Read the model definition and answer for the solid it produces. Units are mm, in the model's axes. A direction names the side the tool comes from. Round coordinates to 2 decimals unless told otherwise and drop trailing zeros. Write each loop counter-clockwise with the first axis right and the second up, starting at its lowest first coordinate (ties: lowest second). Pieces come first, ordered by that corner, then holes. Notation, with made-up numbers: (25, 86.25) - (72, 86.25) arc R22 cw to (72, 93.25) - close; hole circle Ø10 at (8, 76). An arc over 180 degrees is marked (long way). Use one line per item in the form item = value. Start each with the question number.
1) Each of these flat-tipped pins is pushed along its axis until it touches: pin 1 (5 mm diameter, centred on x = -2.5, y = 7, fed in from -Z); pin 2 (0.5 mm diameter, centred on y = -3, z = -9, fed in from -X); pin 3 (2.5 mm diameter, centred on y = 5.5, z = -3.5, fed in from +X). Where does it stop, or does it pass through?
2) The part is cut by section B-B, the plane x = -4. Give the vertices of the cut face in (y, z) (3 decimals), plus the area to 3 significant figures.
3) The part is cut by section A-A, the plane y = -0.25. Give the vertices of the cut face in (x, z), plus the area to 3 significant figures.
4) Consider line 1 along Y through (x, z) = (-4, -1.75) (3 decimals); line 2 along Y through (x, z) = (-4, 2) (3 decimals); line 3 along Y through (x, z) = (-1.25, -9.75). Determine where each line is inside the solid, lowest interval first. Write a range as from..to.
5) For faces 1 (the face through (-4, -2, -11)), 2 (the face through (-4, -2, -1.15)), 3 (the face through (-5.6, 6.7, 2.3)), 4 (the face through (0.4, 1, -9)), 5 (the face through (-4, -2, -1.45)), determine the directions among +Z, -Z, +X, -X, +Y, -Y from which every point of the face is accessible in a straight line to the end or side of a thin tool.
6) For a pull along Z with two mould halves and no side action, classify faces 6 (the face through (0, -2, -9)), 7 (the face through (-4, 2, 0)), 8 (the face through (-4, -2, -10.8)) as released by +Z, released by -Z, zero draft, split by the parting line, or undercut.
7) The part is cut by section C-C, the plane z = 2. Give the vertices of the cut face in (x, y) (3 decimals).
8) The part is cut by section D-D, the plane y = 8. Give the vertices of the cut face in (x, z), plus the area to 3 significant figures.
Autodesk Inventor part; units mm, degrees
ref_plane "YZ Plane" through (0, 0, 0) normal (1, 0, 0) x (0, 1, 0)
ref_plane "XZ Plane" through (0, 0, 0) normal (0, 1, 0) x (-1, 0, 0)
ref_plane "XY Plane" through (0, 0, 0) normal (0, 0, 1) x (1, 0, 0)
sketch "Эскиз1" plane through (0, 0, 0) normal (0, 1, 0) x (-1, 0, 0)
  line L0 (0, 0) -> (8, 0)
  line L1 (8, 0) -> (8, -10.8)
  line L2 (8, -10.8) -> (0, -10.8)
  line L3 (0, -10.8) -> (0, 0)
  dimension "d0" = 10.8
  dimension "d1" = 8
extrude "Выдавливание1" add sketch "Эскиз1" along normal blind 9
sketch "Эскиз2" plane through (-8, 0, 0) normal (0, 0, 1) x (1, 0, 0)
  circle A0 centre (4, 5.5) radius 2.75
  line L0 (8, 0) -> (8, 9)
  line L1 (0, 0) -> (8, 0)
  dimension "d4" = 5.5
  dimension "d5" = 4
  dimension "d6" = 5.5
extrude "Выдавливание2" add sketch "Эскиз2" along normal blind 0.9
sketch "Эскиз3" plane through (-4, 5.5, 0.9) normal (0, 0, 1) x (1, 0, 0)
  circle A0 centre (0, 0) radius 2
  point P0 (4, -5.5)
  dimension "d9" = 4
extrude "Выдавливание3" add sketch "Эскиз3" along normal blind 2.9
sketch "Эскиз4" plane through (-4, 5.5, 3.8) normal (0, 0, 1) x (1, 0, 0)
  circle A0 centre (0, 0) radius 2.75
  circle A1 centre (0, 0) radius 1.275
  point P0 (4, -5.5)
  dimension "d12" = 2.55
extrude "Выдавливание4" cut sketch "Эскиз4" against normal blind 7.9 contours A1
sketch "Эскиз5" plane through (-8, 0, 0) normal (0, 0, 1) x (1, 0, 0)
  point P0 (8, 0)
sketch "Эскиз6" plane through (0, 0, 0) normal (0, -1, 0) x (1, 0, 0)
  line L0 (-4.8, -1.15) -> (-3.2, -1.15)
  line L1 (-3.2, -1.15) -> (-3.2, -1.45)
  line L2 (-3.2, -1.45) -> (-4.8, -1.45)
  line L3 (-4.8, -1.45) -> (-4.8, -1.15)
  line L4 (0, 0) -> (0, -10.8)
  line L5 (-8, 0) -> (0, 0)
  dimension "d15" = 1.6
  dimension "d16" = 0.3
  dimension "d17" = 3.2
  dimension "d18" = 1.15
extrude "Выдавливание5" add sketch "Эскиз6" along normal blind 4
sketch "Эскиз7" plane through (-4.8, 0, -1.15) normal (0, 0, 1) x (1, 0, 0)
  line L0 (0, 0) -> (0, -4)
  line L1 (1.6, 0) -> (1.6, -4)
  arc A0 (0, -3.2011) -> (1.6, -3.2011) centre (0.8, -3.2011) ccw
  line L2 (0, -3.2011) -> (0, -4)
  line L3 (1.6, -4) -> (0, -4)
  line L4 (1.6, -4) -> (1.6, -3.2011)
  point P0 (4.8, 0)
  point P1 (0.7588, -4)
  point P2 (0.8412, -4)
extrude "Выдавливание6" cut sketch "Эскиз7" against normal blind 4
sketch "Эскиз8" plane through (0, 0, 0) normal (1, 0, 0) x (0, 0, -1)
  line L0 (8.2, 5.5) -> (9.8, 5.5)
  line L1 (9.8, 5.5) -> (9.8, -4.5)
  line L2 (9.8, -4.5) -> (8.2, -4.5)
  line L3 (8.2, -4.5) -> (8.2, 5.5)
  line L4 (0, 9) -> (10.8, 9)
  line L5 (0, 0) -> (0, 9)
  dimension "d23" = 1.6
  dimension "d24" = 3.5
  dimension "d25" = 8.2
  dimension "d26" = 10
extrude "Выдавливание7" add sketch "Эскиз8" along normal blind 0.4
sketch "Эскиз9" plane through (0.4, 0, 0) normal (1, 0, 0) x (0, 0, -1)
  line L0 (8.2, 0) -> (8.2, -4.5)
  line L1 (9.8, -4.5) -> (9.8, 0)
  arc A0 (8.2, -3.8439) -> (9.8, -3.8337) centre (8.999, -3.6854) ccw
  line L2 (8.2, -3.8439) -> (8.2, -4.5)
  line L3 (8.2, -4.5) -> (9.8, -4.5)
  line L4 (9.8, -4.5) -> (9.8, -3.8337)
  point P0 (0, 0)
  point P1 (8.9981, -4.5)
extrude "Выдавливание8" cut sketch "Эскиз9" against normal blind 0.4
sketch "Эскиз10" plane through (0, 0, -10.8) normal (0, 0, -1) x (-1, 0, 0)
  line L0 (3, 0.35) -> (5, 0.35)
  line L1 (5, 0.35) -> (5, -4.4)
  line L2 (5, -4.4) -> (3, -4.4)
  line L3 (3, -4.4) -> (3, 0.35)
  line L4 (8, 0) -> (8, 9)
  line L5 (0, 0) -> (8, 0)
  dimension "d31" = 2
  dimension "d32" = 3
  dimension "d33" = 4.75
  dimension "d34" = 0.35
extrude "Выдавливание9" add sketch "Эскиз10" along normal blind 0.2
sketch "Эскиз11" plane through (0, 0, -11) normal (0, 0, -1) x (-1, 0, 0)
  line L0 (3, 0.35) -> (3, -4.4)
  line L1 (5, -4.4) -> (5, 0.35)
  arc A0 (3, -3.4779) -> (5, -3.4779) centre (4, -3.3967) ccw
  line L2 (3, -4.4) -> (5, -4.4)
  line L3 (3, -3.4779) -> (3, -4.4)
  line L4 (3, -4.4) -> (5, -4.4)
  line L5 (5, -4.4) -> (5, -3.4779)
  point P0 (0, 0)
  point P1 (4, -4.4)
extrude "Выдавливание10" cut sketch "Эскиз11" against normal blind 0.2
properties part number "PY-401N"
Geometry results:
q1.pin_1 = -10.8
q1.pin_2 = 0
q1.pin_3 = 0
q2.outline = (-4.4, -11) - (0.35, -11) - (0.35, -10.8) - (9, -10.8) - (9, 0) - (8.25, 0) - (8.25, 0.9) - (7.5, 0.9) - (7.5, 3.8) - (6.775, 3.8) - (6.775, -4.1) - (4.225, -4.1) - (4.225, 3.8) - (3.5, 3.8) - (3.5, 0.9) - (2.75, 0.9) - (2.75, 0) - (0, 0) - (0, -1.15) - (-4.001, -1.15) - (-4.001, -1.45) - (0, -1.45) - (0, -10.8) - (-4.4, -10.8) - close
q2.area = 95.8 mm2
q3.outline = (-5, -11) - (-3, -11) - (-3, -10.8) - (-5, -10.8) - close; (-4.8, -1.45) - (-3.2, -1.45) - (-3.2, -1.15) - (-4.8, -1.15) - close; (0, -9.8) - (0.4, -9.8) - (0.4, -8.2) - (0, -8.2) - close
q3.area = 1.52 mm2
q4.line_1 = 0..4.225, 6.775..9
q4.line_2 = 3.5..4.225, 6.775..7.5
q4.line_3 = 0..9
q5.face_1 = -Z, +X, -X, +Y, -Y
q5.face_2 = +Z, +X, -X, -Y
q5.face_3 = +Z
q5.face_4 = +Z, -Z, +X, +Y, -Y
q5.face_5 = +X, -X, -Y
q6.face_6 = zero draft
q6.face_7 = released by +Z
q6.face_8 = undercut
q7.outline = circle Ø4 at (-4, 5.5); hole circle Ø2.55 at (-4, 5.5)
q8.outline = (-8, -10.8) - (0, -10.8) - (0, 0) - (-2.85, 0) - (-2.85, 0.9) - (-5.15, 0.9) - (-5.15, 0) - (-8, 0) - close
q8.area = 88.5 mm2
